Design review of the part built by this model. Coordinates are the model's own, in mm. A direction names the side the tool comes from. Round coordinates to 2 decimals unless told otherwise and drop trailing zeros. Order: outer loops, then holes, each group sorted by start corner. A loop starts at its lowest first (then second) coordinate and runs counter-clockwise, first axis right, second up. Notation, with made-up numbers: (58.25, -17) - (78.25, -17) arc R13 cw to (78.25, 8) - close; hole circle Ø8 at (23.5, 26). An arc over 180 degrees is marked (long way). Use CSV: the item, a comma, the result in double quotes.
Autodesk Inventor part; units mm, degrees
ref_plane "Work Plane1" through (0, 3, 0) normal (0, 1, 0) x (1, 0, 0)
ref_plane "YZ Plane" through (0, 0, 0) normal (1, 0, 0) x (0, 1, 0)
ref_plane "XZ Plane" through (0, 0, 0) normal (0, 1, 0) x (-1, 0, 0)
sketch "Sketch1" plane through (0, 0, 0) normal (0, 1, 0) x (-1, 0, 0)
  line L0 (-29, 33.75) -> (29, 33.75)
  line L1 (29, 33.75) -> (29, -33.75)
  line L2 (29, -33.75) -> (-29, -33.75)
  line L3 (-29, -33.75) -> (-29, 33.75)
  line L4 (-29, 33.75) -> (29, -33.75) construction
  line L5 (29, 33.75) -> (-29, -33.75) construction
  line L6 (-32.5, 37.25) -> (32.5, 37.25)
  line L7 (32.5, -37.25) -> (-32.5, -37.25)
  line L8 (-32.5, -37.25) -> (-32.5, 37.25)
  line L9 (-32.5, 37.25) -> (32.5, -37.25) construction
  line L10 (32.5, 37.25) -> (-32.5, -37.25) construction
  line L11 (32.5, 37.25) -> (32.5, 5.9791)
  line L12 (32.5, -5.9791) -> (32.5, -37.25)
  line L13 (24.65, -1.5966) -> (24.65, -16)
  circle A0 centre (24.65, -16) radius 1.5
  arc A1 (32.5, 5.9791) -> (32.5, -5.9791) centre (33, 0) ccw
  line L14 (32.5, -5.9791) -> (32.5, 5.9791)
  line L15 (33, 0) -> (-32.5, 0)
  line L16 (24.65, -1.5966) -> (24.65, 16)
  circle A2 centre (24.65, 16) radius 1.5
  circle A3 centre (-18, -33.75) radius 1.5
  circle A4 centre (-18, 33.75) radius 1.5
  point P0 (0, 0)
  dimension "d1" = 58
  dimension "d3" = 3.5
  dimension "d31" = 67.5
  dimension "d32" = 3.5
  dimension "d34" = 3
  dimension "d57" = 47
  dimension "d61" = 42.65
  dimension "d62" = 16
ref_plane "Work Plane1" through (0, 3, 0) normal (0, 1, 0) x (1, 0, 0)
extrude "Extrusion4" add sketch "Sketch1" along normal blind 3 contours A4 L0 L3 L15 L8 L6 L11 A1 L1 | L0 L1 A1 L15 L3 A4 | A1 L1 L2 A3 L3 L15 | L3 L2 A3 L1 A1 L12 L7 L8 L15
sketch "Sketch3" plane through (0, 3, 0) normal (0, 1, 0) x (1, 0, 0)
  circle A0 centre (-24.65, 16) radius 1.5
  circle A1 centre (-24.65, 16) radius 2.85
  circle A2 centre (18, 33.75) radius 1.5
  line L0 (32.5, -37.25) -> (32.5, 37.25)
  line L1 (32.5, 0) -> (-11.5, 0)
  line L2 (-11.5, 0) -> (-11.5, 12.5)
  line L3 (-11.5, 12.5) -> (32.5, 12.5)
  line L4 (32.5, 12.5) -> (32.5, 0)
  line L5 (32.5, 0) -> (32.5, 12.5)
  line L6 (32.5, 0) -> (29, 0)
  line L7 (29, 0) -> (29, 8.825)
  line L8 (29, 8.825) -> (-2, 8.825)
  line L9 (-2, 8.825) -> (-2, 0)
  circle A3 centre (29, 8.825) radius 1
  line L10 (-11.5, 0) -> (-11.5, -12.5)
  line L11 (-11.5, -12.5) -> (32.5, -12.5)
  line L12 (32.5, -12.5) -> (32.5, 0)
  line L13 (29, 0) -> (29, -8.825)
  line L14 (29, -8.825) -> (-2, -8.825)
  line L15 (-2, -8.825) -> (-2, 0)
  circle A4 centre (29, -8.825) radius 1
  line L16 (32.5, 26) -> (32.5, 12.5)
  line L17 (-24.65, 16) -> (-11.5, 12.5)
  line L18 (-25.383, 13.2459) -> (-11.5, 9.5508)
  line L19 (-23.917, 18.7541) -> (-10.0339, 15.059)
  line L20 (32.5, 26) -> (32.5, 12.5)
  line L21 (-10.0339, 15.059) -> (-0.4194, 12.5)
  circle A5 centre (-24.65, -16) radius 2.85
  line L22 (-24.65, -16) -> (-11.5, -12.5)
  line L23 (-25.383, -13.2459) -> (-11.5, -9.5508)
  line L24 (-23.917, -18.7541) -> (-10.0339, -15.059)
  line L25 (-10.0339, -15.059) -> (-0.4194, -12.5)
  circle A6 centre (18, 33.75) radius 2.85
  line L26 (32.5, 12.5) -> (15.5, 12.5)
  circle A7 centre (-2, 6.5) radius 1
  circle A8 centre (-2, -6.5) radius 1
  circle A9 centre (18, 33.75) radius 1.5
  circle A10 centre (18, -33.75) radius 1.5
  circle A11 centre (18, -33.75) radius 2.85
  circle A12 centre (18, -33.75) radius 1.5
  line L27 (20.85, 33.75) -> (20.85, 12.5)
  line L28 (15.15, 33.75) -> (15.15, 12.5)
  line L29 (20.85, -33.75) -> (20.85, -12.5)
  line L30 (15.15, -33.75) -> (15.15, -12.5)
  point P0 (0, 0)
  point P1 (-23.917, 18.7541)
  point P2 (-11.5, -9.5508)
  point P3 (-23.917, -18.7541)
  point P4 (-0.4194, -12.5)
  point P5 (32.5, -12.5)
  point P6 (15.15, -12.5)
  point P7 (20.85, -33.75)
  point P8 (20.85, -12.5)
  point P9 (15.15, 12.5)
  point P10 (20.85, 12.5)
  dimension "d37" = 5.7
  dimension "d38" = 44
  dimension "d39" = 12.5
  dimension "d40" = 3.5
  dimension "d41" = 8.825
  dimension "d42" = 31
  dimension "d44" = 2
  dimension "d48" = 5.7
  dimension "d49" = 17
  dimension "d56" = 6.5
extrude "Extrusion6" cut sketch "Sketch3" against normal blind 44 contours A0 | A1 | A1 L19 L21 L3 L17 | L17 L2 L18 A1 | L3 L0 L1 L7 A3 L8 L9 A7 L2 | L1 L15 A8 L14 A4 L13 L0 L11 L10 | L28 A6 L27 L3 | L9 A7 L8 A3 L7 L1 | L1 L13 A4 L14 L15 A8 | L10 L22 A5 L23 | A6 | L11 L25 L24 A5 L22 | A5 | L11 L29 A11 L30 | A11 | A2 | A10 keep common part
fillet "Fillet3" radius 2 6 edges at (32.5, 1.5, 12.5) (32.5, 1.5, -12.5) (20.85, 1.5, 12.5) (15.15, 1.5, 12.5) (20.85, 1.5, -12.5) (15.15, 1.5, -12.5)
equation "\"d53\" = d38"
properties part number "base_c"
1) The part is to be moulded in two halves that separate along Z. For faces 1 (the face through (19.19, 1.48, 34.66)), 2 (the face through (6, 2, 12.5)), 3 (the face through (15.15, 2, 24)), 4 (the face through (21.45, 1.48, -13.07)), say which applies: +Z half, -Z half, draft (parallel to the pull), parting line (faces both ways), or undercut.
Data:
face 1,"undercut"
face 2,"+Z half"
face 3,"draft"
face 4,"-Z half"
2) We need section C-C (x = -14). Give the boundary of the cut face in (y, z), then the cut area to 3 significant figures.
Data:
outline,"(0, -16.11) - (3, -16.11) - (3, -10.22) - (0, -10.22) - close; (0, 10.22) - (3, 10.22) - (3, 16.11) - (0, 16.11) - close"
area,"35.4 mm2"
3) We need section A-A (z = 6.5). Give the boundary of the cut face in (x, y).
Data:
outline,"(-11.5, 0) - (-3, 0) - (-3, 3) - (-11.5, 3) - close; (-1, 0) - (32.5, 0) - (32.5, 3) - (-1, 3) - close"
4) We need section B-B (x = 18). Give the boundary of the cut face in (y, z), then the cut area to 3 significant figures.
Data:
outline,"(0, -36.6) - (3, -36.6) - (3, -35.25) - (0, -35.25) - close; (0, -32.25) - (3, -32.25) - (3, 32.25) - (0, 32.25) - close; (0, 35.25) - (3, 35.25) - (3, 36.6) - (0, 36.6) - close"
area,"202 mm2"
5) We need section D-D (y = 0.6). Give the number of separate pieces and of enclosed holes in the cut face, then the cut area to 3 significant figures.
Data:
separate pieces,"1"
enclosed holes,"8"
area,"1,540 mm2"
6) For faces 5 (the face through (-18.539, 1.521, -11.424)), 6 (the face through (27, 2, 12.5)), 7 (the face through (14.55, 1.48, 13.07)), 8 (the face through (6, 2, -12.5)), list the 3-axis set-ups (+Z, -Z, +X, -X, +Y, -Y) from which the entire face can be reached by the end or side of a thin tool; tool diameter is ignored.
Data:
face 5,"-X, +Y, -Y"
face 6,"+Z, +X, +Y, -Y"
face 7,"+Z, +Y, -Y"
face 8,"-Z, +Y, -Y"
7) To check wall thickness, follow L1, parallel to Z at x = 18, y = 2.25; L2, parallel to Z at x = 29, y = 1.9 (3 decimals); L3, parallel to Z at x = -24.65, y = 2.35. State the ranges of each line that lie inside material, in increasing order. Write a range as from..to.
Data:
L1,"z = -36.6..-35.25, -32.25..32.25, 35.25..36.6"
L2,"z = -12.5..-9.825, -7.825..7.825, 9.825..12.5"
L3,"z = -18.85..-17.5, -14.5..-13.05, 13.05..14.5, 17.5..18.85"
8) Insertion check: pin 1 Ø1.5 at (x, y) = (-1, 1) entering from +Z; pin 2 Ø0.9 at (x, y) = (25, 2) entering from +Z; pin 3 Ø1 at (x, y) = (-13, 0.5) entering from -Z. Each pin has a flat end and moves straight along its axis. Give the tip position at first contact, or say it passes through.
Data:
pin 1,"stops at z = 12.85"
pin 2,"stops at z = 12.5"
pin 3,"stops at z = -15.98"
